Work out the finished part from the listing and answer in its coordinate system (mm). Face numbers are marked on the shaded views. A direction names the side the tool comes from. Round coordinates to 2 decimals unless told otherwise and drop trailing zeros. Loops run counter-clockwise (first coordinate to the right, second up) from the corner with the lowest first, then second, coordinate; pieces in that order, holes last. Notation, with made-up numbers: (47, 21.25) -> (67, 21.25) arc R10 cw to (67, 28.25) -> close; hole circle Ø1 at (66.5, 63). An arc over 180 degrees is marked (long way). Write item = value, one per line. Start each with the question number.
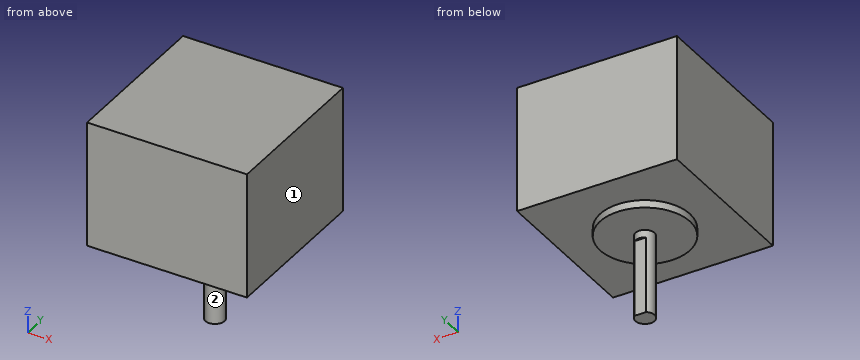
```python
from build123d import *

# Parameters (mm, degrees)
SKETCH1_W           = 42
SKETCH1_H           = 42
BOSS_EXTRUDE1_DEPTH = 33
SKETCH2_R           = 11.793537184
BOSS_EXTRUDE2_DEPTH = 2
SKETCH3_R           = 2.5
BOSS_EXTRUDE3_DEPTH = 22
CUT_EXTRUDE1_DEPTH  = 20


with BuildPart() as part:
    # Sketch1 → Boss-Extrude1 (new body)
    with BuildSketch(Plane.XY):
        Rectangle(SKETCH1_W, SKETCH1_H)
    extrude(amount=BOSS_EXTRUDE1_DEPTH)

    # Sketch2 → Boss-Extrude2 (add)
    with BuildSketch(Plane(origin=(0, 0, 0), x_dir=(-1, 0, 0), z_dir=(0, 0, -1))):
        Circle(SKETCH2_R)
    extrude(amount=BOSS_EXTRUDE2_DEPTH)

    # Sketch3 → Boss-Extrude3 (add)
    with BuildSketch(Plane(origin=(0, 0, -2), x_dir=(-1, 0, 0), z_dir=(0, 0, -1))):
        Circle(SKETCH3_R)
    extrude(amount=BOSS_EXTRUDE3_DEPTH)

    # Sketch4 → Cut-Extrude1 (cut)
    with BuildSketch(Plane(origin=(0, 0, -24), x_dir=(-1, 0, 0), z_dir=(0, 0, -1))):
        with BuildLine():
            Line((1.5, 2), (-1.5, 2))
            ThreePointArc((-1.5, 2), (0, 2.5), (1.5, 2))
        make_face()
    extrude(amount=-CUT_EXTRUDE1_DEPTH, mode=Mode.SUBTRACT)


solid = part.part
```
Item 1: Flat-ended cylindrical pins translate along their axes: pin 1 (1.5 mm diameter, centred on x = 0, z = -16, fed in from +Y); pin 2 (5 mm diameter, centred on x = 13.5, y = -4, fed in from -Z). Find the tip coordinate at first contact, or state that the pin passes through.
Item 2: Find the intervals of material crossed by line 1 along Z through (x, y) = (15.5, 13); line 2 along X through (y, z) = (-1.5, -6.5); line 3 along Y through (x, z) = (0, -13), in increasing order. Write a range as [from, to].
Item 3: Section A-A (x = 0) is taken. Determine the outline of the cut face in (y, z), then the cut area to 3 significant figures.
Item 4: Section C-C (z = -13) is taken. Determine the outline of the cut face in (x, y), then the cut area to 3 significant figures.
Item 5: Section D-D (x = -7) is taken. Determine the outline of the cut face in (y, z), then the cut area to 3 significant figures.
Item 6: Section B-B (y = 0) is taken. Determine the outline of the cut face in (x, z).
Item 7: A tool of negligible diameter and unlimited length cuts with its end or side. For the marked faces 1 and 2, from which of +Z, -Z, +X, -X, +Y, -Y can it reach the whole face along a straight path? Write none if from no direction.
Worked answers:
q1.pin_1 = 2
q1.pin_2 = -2
q2.line_1 = [0, 33]
q2.line_2 = [-2, 2]
q2.line_3 = [-2.5, 2]
q3.outline = (-21, 0) -> (-11.79, 0) -> (-11.79, -2) -> (-2.5, -2) -> (-2.5, -24) -> (2, -24) -> (2, -4) -> (2.5, -4) -> (2.5, -2) -> (11.79, -2) -> (11.79, 0) -> (21, 0) -> (21, 33) -> (-21, 33) -> close
q3.area = 1,530 mm2
q4.outline = (-1.5, 2) arc R2.5 ccw (long way) to (1.5, 2) -> close
q4.area = 18.6 mm2
q5.outline = (-21, 0) -> (-9.49, 0) -> (-9.49, -2) -> (9.49, -2) -> (9.49, 0) -> (21, 0) -> (21, 33) -> (-21, 33) -> close
q5.area = 1,420 mm2
q6.outline = (-21, 0) -> (-11.79, 0) -> (-11.79, -2) -> (-2.5, -2) -> (-2.5, -24) -> (2.5, -24) -> (2.5, -2) -> (11.79, -2) -> (11.79, 0) -> (21, 0) -> (21, 33) -> (-21, 33) -> close
q7.face_1 = +Z, -Z, +X, +Y, -Y
q7.face_2 = -Z
